Can you work these out from the model? Positions are in its coordinate system, mm. A direction names the side the tool comes from. Give positions to 0.01 mm unless a question says otherwise; leave off trailing zeros. Order: outer loops, then holes, each group sorted by start corner. A loop starts at its lowest first (then second) coordinate and runs counter-clockwise, first axis right, second up. Notation, with made-up numbers: (45.5, 71) - (77.5, 71) arc R22 cw to (77.5, 107) - close; hole circle Ø6 at (50, -40). An arc over 180 degrees is marked (long way). Return JSON: item names as keys, results as strings.
```python
from build123d import *

# Parameters (mm, degrees)
F1_DEPTH = 5
F2_SIZE  = 2


# Not quite as in the source:
# - a feature names something its author has since deleted; it is built from what else it names


with BuildPart() as f1:
    # F0 (on Top) → F1 (new body)
    with BuildSketch(Plane.XY):
        with BuildLine():
            ThreePointArc((-64.1, -12.3136591911), (-76.4136591911, 0), (-64.1, 12.3136591911))
            Line((-64.1, 12.3136591911), (0, 12.3136591911))
            Line((0, 12.3136591911), (15.9, 12.3136591911))
            Line((15.9, 12.3136591911), (15.9, 17.3136591911))
            Line((15.9, 17.3136591911), (12.5920902938, 17.3136591911))
            Line((12.5920902938, 17.3136591911), (12.395, 17.3136591911))
            Line((12.395, 17.3136591911), (9.0870902938, 17.3136591911))
            Line((9.0870902938, 17.3136591911), (8.89, 17.3136591911))
            Line((8.89, 17.3136591911), (5.5820902938, 17.3136591911))
            Line((5.5820902938, 17.3136591911), (5.3854580642, 17.3136591911))
            Line((5.3854580642, 17.3136591911), (2.077548358, 17.3136591911))
            Line((2.077548358, 17.3136591911), (1.8804580642, 17.3136591911))
            Line((1.8804580642, 17.3136591911), (0, 17.3136591911))
            Line((0, 17.3136591911), (-1.427451642, 17.3136591911))
            Line((-1.427451642, 17.3136591911), (-1.6245419358, 17.3136591911))
            Line((-1.6245419358, 17.3136591911), (-4.932451642, 17.3136591911))
            Line((-4.932451642, 17.3136591911), (-5.1295419358, 17.3136591911))
            Line((-5.1295419358, 17.3136591911), (-8.437451642, 17.3136591911))
            Line((-8.437451642, 17.3136591911), (-8.6340838715, 17.3136591911))
            Line((-8.6340838715, 17.3136591911), (-11.9419935778, 17.3136591911))
            Line((-11.9419935778, 17.3136591911), (-12.1390838715, 17.3136591911))
            Line((-12.1390838715, 17.3136591911), (-15.4469935778, 17.3136591911))
            Line((-15.4469935778, 17.3136591911), (-15.6440838715, 17.3136591911))
            Line((-15.6440838715, 17.3136591911), (-18.9519935778, 17.3136591911))
            Line((-18.9519935778, 17.3136591911), (-19.1490838715, 17.3136591911))
            Line((-19.1490838715, 17.3136591911), (-22.4569935778, 17.3136591911))
            Line((-22.4569935778, 17.3136591911), (-22.6536258073, 17.3136591911))
            Line((-22.6536258073, 17.3136591911), (-25.9615355136, 17.3136591911))
            Line((-25.9615355136, 17.3136591911), (-64.1, 17.3136591911))
            ThreePointArc((-64.1, 17.3136591911), (-81.4136591911, 0), (-64.1, -17.3136591911))
            Line((-64.1, -17.3136591911), (0, -17.3136591911))
            Line((0, -17.3136591911), (15.9, -17.3136591911))
            Line((15.9, -17.3136591911), (15.9, -12.3136591911))
            Line((15.9, -12.3136591911), (0, -12.3136591911))
            Line((0, -12.3136591911), (-64.1, -12.3136591911))
        make_face()
        Polygon((12.5920902938, 17.3136591911), (15.9, 17.3136591911), (12.5920902938, 22.3136591911), align=None)
        Polygon((9.0870902938, 17.3136591911), (12.395, 17.3136591911), (9.0870902938, 22.3136591911), align=None)
        Polygon((5.5820902938, 17.3136591911), (8.89, 17.3136591911), (5.5820902938, 22.3136591911), align=None)
        Polygon((2.077548358, 17.3136591911), (5.3854580642, 17.3136591911), (2.077548358, 22.3136591911), align=None)
        Polygon((0, 17.3136591911), (1.8804580642, 17.3136591911), (-1.427451642, 22.3136591911), (-1.427451642, 17.3136591911), align=None)
        Polygon((-4.932451642, 17.3136591911), (-1.6245419358, 17.3136591911), (-4.932451642, 22.3136591911), align=None)
        Polygon((-8.437451642, 17.3136591911), (-5.1295419358, 17.3136591911), (-8.437451642, 22.3136591911), align=None)
        Polygon((-11.9419935778, 22.3136591911), (-11.9419935778, 17.3136591911), (-8.6340838715, 17.3136591911), align=None)
        Polygon((-15.4469935778, 22.3136591911), (-15.4469935778, 17.3136591911), (-12.1390838715, 17.3136591911), align=None)
        Polygon((-18.9519935778, 22.3136591911), (-18.9519935778, 17.3136591911), (-15.6440838715, 17.3136591911), align=None)
        Polygon((-22.4569935778, 22.3136591911), (-22.4569935778, 17.3136591911), (-19.1490838715, 17.3136591911), align=None)
        Polygon((-25.9615355136, 22.3136591911), (-25.9615355136, 17.3136591911), (-22.6536258073, 17.3136591911), align=None)
    extrude(amount=F1_DEPTH)

    # F2
    f2_edges = [f1.edges().sort_by_distance(p)[0] for p in [
        (-76.413659, 0, 5),
        (-76.413659, 0, 0),
    ]]
    chamfer(f2_edges, length=F2_SIZE)


solid = f1.part
```
1. Thinking about a two-plate mould opening in Y: for faces 4 (the face through (2.078, 20, 2)), 5 (the face through (-24.66, 13.328, 0.986)), 6 (the face through (-81.41, 0.38, 2.46)), which applies, +Y half, -Y half, draft (parallel to the pull), parting line (faces both ways), or undercut?
Checks:
{"face 4": "draft", "face 5": "undercut", "face 6": "parting line"}
2. For pin 1 Ø2.5 at (y, z) = (20, 1.5) entering from -X; pin 2 Ø1 at (x, z) = (-7.5, 2.5) entering from +Y; pin 3 Ø1 at (y, z) = (-2.5, 1.5) entering from +X; pin 4 Ø10 at (x, y) = (-27.5, 7) entering from -Z, each with a flat end and sliding along its axis, tell me the tip position at first contact or that it passes through.
Checks:
{"pin 1": "x = -25.96", "pin 2": "y = 21.65", "pin 3": "x = -76.15", "pin 4": "through"}
3. If I drill on L1, parallel to Y at x = -65, z = 4.65; L2, parallel to Y at x = -57, z = 4.25; L3, parallel to X at y = -0.5, z = 2.9, over which ranges is the centre line in solid material (lowest first)? Write a range as [from, to].
Checks:
{"L1": "[-17.29, -13.93], [13.93, 17.29]", "L2": "[-17.31, -13.56], [13.56, 17.31]", "L3": "[-81.41, -76.4]"}
4. Suppose I cut it at A-A (x = -39). List the corners of the cut face in (y, z) for me, plus the area to 3 significant figures.
Checks:
{"outline": "(-17.31, 0) - (-14.31, 0) - (-12.31, 2) - (-12.31, 3) - (-14.31, 5) - (-17.31, 5) - close; (12.31, 2) - (14.31, 0) - (17.31, 0) - (17.31, 5) - (14.31, 5) - (12.31, 3) - close", "area": "42.0 mm^2"}
5. Suppose I cut it at B-B (y = 0). List the corners of the cut face in (x, z) for me.
Checks:
{"outline": "(-81.41, 0) - (-78.41, 0) - (-76.41, 2) - (-76.41, 3) - (-78.41, 5) - (-81.41, 5) - close"}
6. On a 3-axis mill with a long thin cutter (end or side, diameter ignored), from which of +Z, -Z, +X, -X, +Y, -Y can I reach the whole of each face in a straight line? I mean faces 1 (the face through (-23.54, -13.328, 0.986)), 2 (the face through (-25.962, 20, 2)), 3 (the face through (-10.265, 19.779, 2.465)). Say none if no direction works.
Checks:
{"face 1": "-Z, +X", "face 2": "+Z, -Z, -X, +Y", "face 3": "+Z, -Z, +Y"}
7. Suppose I cut it at C-C (x = -18). List the corners of the cut face in (y, z) for me.
Checks:
{"outline": "(-17.31, 0) - (-14.31, 0) - (-12.31, 2) - (-12.31, 3) - (-14.31, 5) - (-17.31, 5) - close; (12.31, 2) - (14.31, 0) - (20.87, 0) - (20.87, 5) - (14.31, 5) - (12.31, 3) - close"}
